The model under review builds one solid part; all positions refer to its coordinate system, in mm. A direction names the side the tool comes from. Give positions to 0.01 mm unless a question says otherwise; leave off trailing zeros. Order: outer loops, then holes, each group sorted by start corner. A loop starts at its lowest first (then second) coordinate and runs counter-clockwise, first axis right, second up.
```python
from build123d import *

# Parameters (mm, degrees)
BOSS_EXTRUDE1_DEPTH = 1
BOSS_EXTRUDE2_DEPTH = 1.25


with BuildPart() as part:
    # Sketch1 → Boss-Extrude1 (new body)
    with BuildSketch(Plane(origin=(0, 0, 0), x_dir=(0, 0, -1), z_dir=(1, 0, 0))):
        with BuildLine():
            ThreePointArc((3, 0), (0, 3), (-3, 0))
            Line((-3, 0), (-1.2, 0))
            ThreePointArc((-1.2, 0), (0, 1.2), (1.2, 0))
            Line((1.2, 0), (3, 0))
        make_face()
        with BuildLine():
            ThreePointArc((1.2, 0), (0, 1.2), (-1.2, 0))
            Line((-1.2, 0), (1.2, 0))
        make_face()
    extrude(amount=BOSS_EXTRUDE1_DEPTH)

    # Sketch1_3 → Boss-Extrude2 (add)
    with BuildSketch(Plane(origin=(0, 0, 0), x_dir=(0, 0, -1), z_dir=(1, 0, 0))):
        with BuildLine():
            ThreePointArc((1.2, 0), (0, 1.2), (-1.2, 0))
            Line((-1.2, 0), (1.2, 0))
        make_face()
    extrude(amount=-BOSS_EXTRUDE2_DEPTH)

    # Mirror1: part across plane


with BuildPart() as part_1:
    add(part.part)
    add(part.part.mirror(Plane.ZY.offset(1.25)))


solid = part_1.part
```
Item 1: Take a section at C-C (z = 2.45). Give the boundary of the cut face in (x, y).
Values found:
outline: (-3.5, 0) - (-2.5, 0) - (-2.5, 1.73) - (-3.5, 1.73) - close; (0, 0) - (1, 0) - (1, 1.73) - (0, 1.73) - close
Item 2: Take a section at D-D (x = -3.1). Give the boundary of the cut face in (y, z).
Values found:
outline: (0, -3) arc R3 ccw to (0, 3) - close
Item 3: For faces 1 (the cylindrical face through (-1.3, 1.2, 0)), 2 (the flat face through (-3.5, 1, 0)), list the 3-axis set-ups (+Z, -Z, +X, -X, +Y, -Y) from which the entire face can be reached by the end or side of a thin tool; tool diameter is ignored.
Values found:
face 1: +Y
face 2: +Z, -Z, -X, +Y, -Y
Item 4: Take a section at B-B (z = 0). Give the boundary of the cut face in (x, y).
Values found:
outline: (-3.5, 0) - (1, 0) - (1, 3) - (0, 3) - (0, 1.2) - (-2.5, 1.2) - (-2.5, 3) - (-3.5, 3) - close
Item 5: Take a section at A-A (y = 1.8). Give the boundary of the cut face in (x, z), and give its area (3 significant figures).
Values found:
outline: (-3.5, -2.4) - (-2.5, -2.4) - (-2.5, 2.4) - (-3.5, 2.4) - close; (0, -2.4) - (1, -2.4) - (1, 2.4) - (0, 2.4) - close
area: 9.60 mm2
Item 6: Draft analysis for pull direction X (two halves, no side actions). For faces 3 (the flat face through (0, 2, 0)), 4 (the flat face through (1, 1, 0)), 5 (the cylindrical face through (-3, 3, 0)), 6 (the flat face through (-2.5, 2, 0)), state which applies: released by +X, released by -X, zero draft, split by the parting line, or undercut.
Values found:
face 3: undercut
face 4: released by +X
face 5: zero draft
face 6: undercut
Item 7: For line 1 (X direction, y = 2.7, z = -1.05); line 2 (Z direction, x = 0.7, y = 1.6); line 3 (Z direction, x = 0.45, y = 1.9), list the stretches that pass through material, from the lowest coordinate up.
Values found:
line 1: x = -3.5 to -2.5, 0 to 1
line 2: z = -2.54 to 2.54
line 3: z = -2.32 to 2.32
